```python
from build123d import *

# Parameters (mm, degrees)
SKETCH1_R             = 3.25
SKETCH1_R_2           = 1.65
BOSS_EXTRUDE1_DEPTH   = 6
BOSS_EXTRUDE1_2_DEPTH = 6
BOSS_EXTRUDE1_3_DEPTH = 6
BOSS_EXTRUDE1_4_DEPTH = 6
SKETCH2_W             = 45
SKETCH2_H             = 45
BOSS_EXTRUDE2_DEPTH   = 3
CUT_EXTRUDE1_START    = -3
SKETCH1_2_R           = 1.65
CUT_EXTRUDE1_DEPTH    = 3
SKETCH7_W             = 9.5
SKETCH7_H             = 45
BOSS_EXTRUDE3_DEPTH   = 25
SKETCH8_R             = 2.5
CUT_EXTRUDE2_DEPTH    = 58.578207683


with BuildPart() as part:
    # Sketch1 → Boss-Extrude1 (new body)
    with BuildSketch(Plane(origin=(0, 0, 0), x_dir=(1, 0, 0), z_dir=(0, 1, 0))):
        with Locations(Location((-15.25, 15.25, 0), (0, 0, 270))):
            Circle(SKETCH1_R)
        with Locations(Location((-15.25, 15.25, 0), (0, 0, 270))):
            Circle(SKETCH1_R_2, mode=Mode.SUBTRACT)
    extrude(amount=BOSS_EXTRUDE1_DEPTH)



with BuildPart() as body_2:
    # Sketch1 → Boss-Extrude1 2 (new body)
    with BuildSketch(Plane(origin=(0, 0, 0), x_dir=(1, 0, 0), z_dir=(0, 1, 0))):
        with Locations(Location((15.25, 15.25, 0), (0, 0, 270))):
            Circle(SKETCH1_R)
        with Locations(Location((15.25, 15.25, 0), (0, 0, 270))):
            Circle(SKETCH1_R_2, mode=Mode.SUBTRACT)
    extrude(amount=BOSS_EXTRUDE1_2_DEPTH)


with BuildPart() as body_3:
    # Sketch1 → Boss-Extrude1 3 (new body)
    with BuildSketch(Plane(origin=(0, 0, 0), x_dir=(1, 0, 0), z_dir=(0, 1, 0))):
        with Locations(Location((15.25, -15.25, 0), (0, 0, 270))):
            Circle(SKETCH1_R)
        with Locations(Location((15.25, -15.25, 0), (0, 0, 270))):
            Circle(SKETCH1_R_2, mode=Mode.SUBTRACT)
    extrude(amount=BOSS_EXTRUDE1_3_DEPTH)


with BuildPart() as body_4:
    # Sketch1 → Boss-Extrude1 4 (new body)
    with BuildSketch(Plane(origin=(0, 0, 0), x_dir=(1, 0, 0), z_dir=(0, 1, 0))):
        with Locations(Location((-15.25, -15.25, 0), (0, 0, 270))):
            Circle(SKETCH1_R)
        with Locations(Location((-15.25, -15.25, 0), (0, 0, 270))):
            Circle(SKETCH1_R_2, mode=Mode.SUBTRACT)
    extrude(amount=BOSS_EXTRUDE1_4_DEPTH)


with BuildPart() as part_1:
    add(part.part)

    add(body_2.part)  # Boss-Extrude2 merges body 2

    add(body_3.part)  # Boss-Extrude2 merges body 3

    add(body_4.part)  # Boss-Extrude2 merges body 4
    # Sketch2 → Boss-Extrude2 (add)
    with BuildSketch(Plane(origin=(0, 0, 0), x_dir=(1, 0, 0), z_dir=(0, 1, 0))):
        Rectangle(SKETCH2_W, SKETCH2_H)
    extrude(amount=-BOSS_EXTRUDE2_DEPTH)

    # Sketch1_2 → Cut-Extrude1 (cut)
    with BuildSketch(Plane(origin=(0, 0, 0), x_dir=(1, 0, 0), z_dir=(0, 1, 0)).offset(CUT_EXTRUDE1_START)):
        with Locations(Location((-15.25, 15.25, 0), (0, 0, 270))):
            Circle(SKETCH1_2_R)
        with Locations(Location((-15.25, -15.25, 0), (0, 0, 270))):
            Circle(SKETCH1_2_R)
        with Locations(Location((15.25, -15.25, 0), (0, 0, 270))):
            Circle(SKETCH1_2_R)
        with Locations(Location((15.25, 15.25, 0), (0, 0, 270))):
            Circle(SKETCH1_2_R)
    extrude(amount=CUT_EXTRUDE1_DEPTH, mode=Mode.SUBTRACT)

    # Sketch7 → Boss-Extrude3 (add)
    with BuildSketch(Plane.XZ.offset(3)):
        with Locations((-17.75, 0)):
            Rectangle(SKETCH7_W, SKETCH7_H)
        with Locations((17.75, 0)):
            Rectangle(SKETCH7_W, SKETCH7_H)
    extrude(amount=BOSS_EXTRUDE3_DEPTH)

    # Sketch8 → Cut-Extrude2 (cut, through all)
    with BuildSketch(Plane(origin=(22.5, 0, 0), x_dir=(0, 0, -1), z_dir=(1, 0, 0))):
        with Locations((0, -14)):
            Circle(SKETCH8_R)
        with Locations((-10, -14)):
            Circle(SKETCH8_R)
        with Locations((10, -14)):
            Circle(SKETCH8_R)
    extrude(amount=-CUT_EXTRUDE2_DEPTH, mode=Mode.SUBTRACT)


solid = part_1.part
```
Design review of the part built by this model. Coordinates are the model's own, in mm. A direction names the side the tool comes from. Round coordinates to 2 decimals unless told otherwise and drop trailing zeros. Write each loop counter-clockwise with the first axis right and the second up, starting at its lowest first coordinate (ties: lowest second). Pieces come first, ordered by that corner, then holes. Notation, with made-up numbers: (56.5, 89.25) -> (88.5, 89.25) arc R25 ccw to (88.5, 105.25) -> close; hole circle Ø7 at (47.25, 44). An arc over 180 degrees is marked (long way). Write item = value, one per line. Start each with the question number.
1) Wall thickness on probe 1 along Y at (x, z) = (-20.5, 10); probe 2 along X at (y, z) = (-20.5, -17.5); probe 3 along Z at (x, y) = (-18.5, -15): over which ranges is each line inside the solid? List them lowest first. Write a range as from..to.
2) Take a section at D-D, the plane y = -20. State the section outline as (x, z) points.
3) Take a section at C-C, the plane x = 15.25. State the section outline as (y, z) points, plus the area to 3 significant figures.
4) Tool access review of faces 5 (the face through (-17.7, -15.5, 12)), 6 (the face through (-12.028, 2.958, -15.673)), 7 (the face through (-13, -18, 0)): name each direction out of +Z, -Z, +X, -X, +Y, -Y from which nothing blocks a thin tool from reaching the whole face with its end or side.
5) Clearance check with flat-ended pins moving along their axes: pin 1 (4 mm diameter, centred on y = -14, z = 10, fed in from -X); pin 2 (1 mm diameter, centred on x = -2.5, z = 15, fed in from +Y); pin 3 (1.6 mm diameter, centred on x = 14.5, z = 15, fed in from +Y). State where each tip first meets the part, or that it passes through.
6) Take a section at A-A, the plane z = 0. State the section outline as (x, y) points.
7) Take a section at B-B, the plane y = -15.5. Count the separate pieces of the cut face and the enclosed holes in it, plus the area to 3 significant figures.
8) Mouldability with a two-part tool opening along X and no side actions: class faces 1 (the face through (-17.68, -16.44, 0.54)), 2 (the face through (22.5, -11, 0)), 3 (the face through (0, 0, 0)), 4 (the face through (-14.754, 1.437, 16.824)) as +X half, -X half, draft (parallel to the pull), parting line (faces both ways), or undercut.
Results list:
q1.probe_1 = -28..-16.5, -11.5..0
q1.probe_2 = -22.5..-13, 13..22.5
q1.probe_3 = -22.5..-12.29, -7.71..-2.29, 2.29..7.71, 12.29..22.5
q2.outline = (-22.5, -22.5) -> (-13, -22.5) -> (-13, 22.5) -> (-22.5, 22.5) -> close; (13, -22.5) -> (22.5, -22.5) -> (22.5, 22.5) -> (13, 22.5) -> close
q3.outline = (-28, -22.5) -> (0, -22.5) -> (0, -18.5) -> (6, -18.5) -> (6, -16.9) -> (-3, -16.9) -> (-3, -13.6) -> (6, -13.6) -> (6, -12) -> (0, -12) -> (0, 12) -> (6, 12) -> (6, 13.6) -> (-3, 13.6) -> (-3, 16.9) -> (6, 16.9) -> (6, 18.5) -> (0, 18.5) -> (0, 22.5) -> (-28, 22.5) -> close; hole circle Ø5 at (-14, -10); hole circle Ø5 at (-14, 0); hole circle Ø5 at (-14, 10)
q3.area = 1,220 mm²
q4.face_5 = +X, -X
q4.face_6 = +Y
q4.face_7 = +Z, -Z, -Y
q5.pin_1 = through
q5.pin_2 = 0
q5.pin_3 = -3
q6.outline = (-22.5, -28) -> (-13, -28) -> (-13, -16.5) -> (-22.5, -16.5) -> close; (-22.5, -11.5) -> (-13, -11.5) -> (-13, -3) -> (13, -3) -> (13, -11.5) -> (22.5, -11.5) -> (22.5, 0) -> (-22.5, 0) -> close; (13, -28) -> (22.5, -28) -> (22.5, -16.5) -> (13, -16.5) -> close
q7.separate_pieces = 8
q7.enclosed_holes = 0
q7.area = 627 mm²
q8.face_1 = draft
q8.face_2 = +X half
q8.face_3 = undercut
q8.face_4 = undercut
